```python
from build123d import *

# Parameters (mm, degrees)
SKETCH1_W           = 40
SKETCH1_H           = 30
BOSS_EXTRUDE1_DEPTH = 5
SKETCH2_W           = 40
SKETCH2_H           = 5
BOSS_EXTRUDE2_DEPTH = 45.5
SKETCH3_W           = 57.5
SKETCH3_H           = 5
BOSS_EXTRUDE3_DEPTH = 5
FILLET1_R           = 10
FILLET2_R           = 5
FILLET3_R           = 10
SKETCH4_R           = 3
CUT_EXTRUDE1_DEPTH  = 86.36099812


with BuildPart() as part:
    # Sketch1 → Boss-Extrude1 (new body)
    with BuildSketch(Plane(origin=(0, 0, 0), x_dir=(1, 0, 0), z_dir=(0, 1, 0))):
        with Locations((37.5, 15)):
            Rectangle(SKETCH1_W, SKETCH1_H)
    extrude(amount=BOSS_EXTRUDE1_DEPTH)

    # Sketch2 → Boss-Extrude2 (add)
    with BuildSketch(Plane.XZ):
        with Locations((37.5, -2.5)):
            Rectangle(SKETCH2_W, SKETCH2_H)
    extrude(amount=BOSS_EXTRUDE2_DEPTH)

    # Sketch3 → Boss-Extrude3 (add)
    with BuildSketch(Plane.XZ.offset(45.5)):
        with Locations((28.75, -2.5)):
            Rectangle(SKETCH3_W, SKETCH3_H)
    extrude(amount=BOSS_EXTRUDE3_DEPTH)

    # Fillet1
    fillet1_edges = [part.edges().sort_by_distance(p)[0] for p in [
        (57.5, -50.5, -2.5),
    ]]
    fillet(fillet1_edges, radius=FILLET1_R)

    # Fillet2
    fillet2_edges = [part.edges().sort_by_distance(p)[0] for p in [
        (17.5, -45.5, -2.5),
    ]]
    fillet(fillet2_edges, radius=FILLET2_R)

    # Fillet3
    fillet3_edges = [part.edges().sort_by_distance(p)[0] for p in [
        (17.5, 2.5, -30),
        (57.5, 2.5, -30),
    ]]
    fillet(fillet3_edges, radius=FILLET3_R)

    # Sketch4 → Cut-Extrude1 (cut, through all)
    with BuildSketch(Plane(origin=(0, 5, 0), x_dir=(1, 0, 0), z_dir=(0, 1, 0))):
        with Locations(Location((37.5, 22, 0), (0, 0, 270))):
            Circle(SKETCH4_R)
    extrude(amount=-CUT_EXTRUDE1_DEPTH, mode=Mode.SUBTRACT)

    # Mirror1: part across plane


with BuildPart() as part_1:
    add(part.part)
    add(part.part.mirror(Plane(origin=(0, 0, 0), x_dir=(0, 0, 1), z_dir=(1, 0, 0))))


solid = part_1.part
```
Read the model definition and answer for the solid it produces. Units are mm, in the model's axes. A direction names the side the tool comes from. Give positions to 0.01 mm unless a question says otherwise; leave off trailing zeros. Write each loop counter-clockwise with the first axis right and the second up, starting at its lowest first coordinate (ties: lowest second). Pieces come first, ordered by that corner, then holes. Notation, with made-up numbers: (-6, 16) -> (50, 16) arc R13 ccw to (50, 27) -> close; hole circle Ø7 at (50, -30). An arc over 180 degrees is marked (long way). Answer in a Markdown table with one row per item.
1) Section B-B on y = -10 is taken. Give the vertices of the cut face in (x, z), plus the area to 3 significant figures.
Results list:
| item | result |
|---|---|
| outline | (-57.5, -5) -> (-17.5, -5) -> (-17.5, 0) -> (-57.5, 0) -> close; (17.5, -5) -> (57.5, -5) -> (57.5, 0) -> (17.5, 0) -> close |
| area | 400 mm^2 |
2) Section C-C on x = 37.5 is taken. Give the vertices of the cut face in (y, z).
Results list:
| item | result |
|---|---|
| outline | (-50.5, -5) -> (0, -5) -> (0, -19) -> (5, -19) -> (5, 0) -> (-50.5, 0) -> close; (0, -30) -> (5, -30) -> (5, -25) -> (0, -25) -> close |
3) Each of these flat-tipped pins is pushed along its axis until it touches: pin 1 Ø3 at (x, z) = (20.5, -17) entering from -Y; pin 2 Ø3 at (x, z) = (-7.5, -8) entering from +Y; pin 3 Ø2.5 at (x, z) = (-2.5, -2) entering from +Y. Where does it stop, or does it pass through?
Results list:
| item | result |
|---|---|
| pin 1 | y = 0 |
| pin 2 | through |
| pin 3 | y = -45.5 |
4) Straight lines are drawn through the part: line 1 (X direction, y = 1.15, z = -22); line 2 (Y direction, x = -26, z = -12); line 3 (Z direction, x = 38, y = -34). For each, find the intervals that lie inside material, in ascending order. Write a range as [from, to].
Results list:
| item | result |
|---|---|
| line 1 | [-57.3, -40.5], [-34.5, -17.7], [17.7, 34.5], [40.5, 57.3] |
| line 2 | [0, 5] |
| line 3 | [-5, 0] |
5) A tool of negligible diameter and unlimited length cuts with its end or side. For faces 1 (the flat face through (1, -47, -5)), 2 (the cylindrical face through (-20.35, 2.54, -26.99)), 3 (the cylindrical face through (-54.49, -47.65, -2.46)), 4 (the cylindrical face through (-16, -44.07, -2.46)), from which of +Z, -Z, +X, -X, +Y, -Y can it reach the whole face along a straight path? Write none if from no direction.
Results list:
| item | result |
|---|---|
| face 1 | -Z, +X, -X, -Y |
| face 2 | -Z, +Y, -Y |
| face 3 | +Z, -Z, -X, -Y |
| face 4 | +Z, -Z, +Y |
6) Section A-A on z = -11 is taken. Give the vertices of the cut face in (x, y).
Results list:
| item | result |
|---|---|
| outline | (-57.5, 0) -> (-17.5, 0) -> (-17.5, 5) -> (-57.5, 5) -> close; (17.5, 0) -> (57.5, 0) -> (57.5, 5) -> (17.5, 5) -> close |
7) Determine the mould class of faces 5 (the flat face through (-57.5, -13, -4)), 6 (the flat face through (1, -50.5, -2)), 7 (the flat face through (0, -45.5, -2)) for opening direction X: released by +X, released by -X, zero draft, split by the parting line, or undercut.
Results list:
| item | result |
|---|---|
| face 5 | released by -X |
| face 6 | zero draft |
| face 7 | undercut |
8) Section D-D on z = -22 is taken. Give the vertices of the cut face in (x, y).
Results list:
| item | result |
|---|---|
| outline | (-57.3, 0) -> (-40.5, 0) -> (-40.5, 5) -> (-57.3, 5) -> close; (-34.5, 0) -> (-17.7, 0) -> (-17.7, 5) -> (-34.5, 5) -> close; (17.7, 0) -> (34.5, 0) -> (34.5, 5) -> (17.7, 5) -> close; (40.5, 0) -> (57.3, 0) -> (57.3, 5) -> (40.5, 5) -> close |
